Source: CAD feature listing. Evaluate the final solid. Frame: model axes, mm. A direction names the side the tool comes from. Coordinates: 2 decimals unless noted, no trailing zeros. Write each loop counter-clockwise with the first axis right and the second up, starting at its lowest first coordinate (ties: lowest second). Pieces come first, ordered by that corner, then holes. Notation, with made-up numbers: M -31.75,27.25 L 9.25,27.25 A17 cw 9.25,52.25 Z; hole C 66.25,-40 d6. An arc over 180 degrees is marked long. Write item = value, one per line. Start each with the question number.
1. Pull-direction query (X, two-part tool) for faces 4 (the face through (-110, 4, 2)), 5 (the face through (102, 16, 2)), 6 (the face through (77.5, 72, 2)), 7 (the face through (87.5, 72, 2)); classes: pulls with the +X half, pulls with the -X half, needs draft (parallel to the pull), parting line crosses it, or undercut.
2. Access query for faces 1 (the face through (-110, 71, 2)), 2 (the face through (17.5, -2, 2)), 3 (the face through (-35, 70, 2)). Directions: +Z, -Z, +X, -X, +Y, -Y. A direction counts if a zero-diameter tool reaches every point of the face in a straight line with its end or side. Return the directions, or none.
3. Pin query (flat end, axial travel): pin 1 Ø2.5 at (y, z) = (-3.5, 1.5) entering from -X; pin 2 Ø1.5 at (y, z) = (30.5, 2) entering from -X; pin 3 Ø1.5 at (x, z) = (-83, 0.5) entering from -Y; pin 4 Ø12 at (x, y) = (-53, 52.5) entering from -Z. Return the tip coordinate at first contact, or that it passes through.
4. Line query: line 1 along X through (y, z) = (4, 4.45); line 2 along X through (y, z) = (55, 3); line 3 along Y through (x, z) = (82.5, 2.05). Output: solid intervals per line, ascending.
5. Section query A-A (x = 4). Output: boundary loops of the cut face in (y, z).
6. Section query B-B (z = 1.75). Give the number of separate pieces and of enclosed holes in the cut face, then the cut area to 3 significant figures.
```python
from build123d import *

# Parameters (mm, degrees)
SKETCH1_W           = 5
SKETCH1_H           = 5
SKETCH1_R           = 1.5
BOSS_EXTRUDE2_DEPTH = 5


with BuildPart() as part:
    # Sketch1 → Boss-Extrude2 (new body)
    with BuildSketch(Plane.XY):
        Polygon((-110, 80), (-110, 62.5), (-115, 62.5), (-115, 57.5), (-110, 57.5), (-110, 54), (-107, 54), (-107, 55.1), (-104.7, 55.1), (-104.7, 54), (-100, 54), (-100, 51), (-104.7, 51), (-104.7, 49.9), (-107, 49.9), (-107, 51), (-110, 51), (-110, 47.5), (-115, 47.5), (-115, 42.5), (-110, 42.5), (-110, 27.5), (-115, 27.5), (-115, 22.5), (-110, 22.5), (-110, 19), (-107, 19), (-107, 20.1), (-104.7, 20.1), (-104.7, 19), (-100, 19), (-100, 16), (-104.7, 16), (-104.7, 14.9), (-107, 14.9), (-107, 16), (-110, 16), (-110, 12.5), (-115, 12.5), (-115, 7.5), (-110, 7.5), (-110, 0), (-92.5, 0), (-92.5, -5), (-87.5, -5), (-87.5, 0), (-84, 0), (-84, 3), (-85.1, 3), (-85.1, 5.3), (-84, 5.3), (-84, 10), (-81, 10), (-81, 5.3), (-79.9, 5.3), (-79.9, 3), (-81, 3), (-81, 0), (-77.5, 0), (-77.5, -5), (-72.5, -5), (-72.5, 0), (-37.5, 0), (-37.5, -5), (-32.5, -5), (-32.5, 0), (-29, 0), (-29, 3), (-30.1, 3), (-30.1, 5.3), (-29, 5.3), (-29, 10), (-26, 10), (-26, 5.3), (-24.9, 5.3), (-24.9, 3), (-26, 3), (-26, 0), (-22.5, 0), (-22.5, -5), (-17.5, -5), (-17.5, 0), (17.5, 0), (17.5, -5), (22.5, -5), (22.5, 0), (26, 0), (26, 3), (24.9, 3), (24.9, 5.3), (26, 5.3), (26, 10), (29, 10), (29, 5.3), (30.1, 5.3), (30.1, 3), (29, 3), (29, 0), (32.5, 0), (32.5, -5), (37.5, -5), (37.5, 0), (72.5, 0), (72.5, -5), (77.5, -5), (77.5, 0), (81, 0), (81, 3), (79.9, 3), (79.9, 5.3), (81, 5.3), (81, 10), (84, 10), (84, 5.3), (85.1, 5.3), (85.1, 3), (84, 3), (84, 0), (87.5, 0), (87.5, -5), (92.5, -5), (92.5, 0), (110, 0), (110, 7.5), (115, 7.5), (115, 12.5), (110, 12.5), (110, 16), (107, 16), (107, 14.9), (104.7, 14.9), (104.7, 16), (100, 16), (100, 19), (104.7, 19), (104.7, 20.1), (107, 20.1), (107, 19), (110, 19), (110, 22.5), (115, 22.5), (115, 27.5), (110, 27.5), (110, 42.5), (115, 42.5), (115, 47.5), (110, 47.5), (110, 51), (107, 51), (107, 49.9), (104.7, 49.9), (104.7, 51), (100, 51), (100, 54), (104.7, 54), (104.7, 55.1), (107, 55.1), (107, 54), (110, 54), (110, 57.5), (115, 57.5), (115, 62.5), (110, 62.5), (110, 80), align=None)
        with Locations((-90, 72.5)):
            Rectangle(SKETCH1_W, SKETCH1_H, mode=Mode.SUBTRACT)
        with Locations((-82.5, 72.5)):
            Circle(SKETCH1_R, mode=Mode.SUBTRACT)
        with Locations((-75, 72.5)):
            Rectangle(SKETCH1_W, SKETCH1_H, mode=Mode.SUBTRACT)
        with Locations((-35, 72.5)):
            Rectangle(SKETCH1_W, SKETCH1_H, mode=Mode.SUBTRACT)
        with Locations((-27.5, 72.5)):
            Circle(SKETCH1_R, mode=Mode.SUBTRACT)
        with Locations((-20, 72.5)):
            Rectangle(SKETCH1_W, SKETCH1_H, mode=Mode.SUBTRACT)
        with Locations((20, 72.5)):
            Rectangle(SKETCH1_W, SKETCH1_H, mode=Mode.SUBTRACT)
        with Locations((27.5, 72.5)):
            Circle(SKETCH1_R, mode=Mode.SUBTRACT)
        with Locations((35, 72.5)):
            Rectangle(SKETCH1_W, SKETCH1_H, mode=Mode.SUBTRACT)
        with Locations((75, 72.5)):
            Rectangle(SKETCH1_W, SKETCH1_H, mode=Mode.SUBTRACT)
        with Locations((82.5, 72.5)):
            Circle(SKETCH1_R, mode=Mode.SUBTRACT)
        with Locations((90, 72.5)):
            Rectangle(SKETCH1_W, SKETCH1_H, mode=Mode.SUBTRACT)
    extrude(amount=BOSS_EXTRUDE2_DEPTH)


solid = part.part
```
Results are:
q1.face_4 = pulls with the -X half
q1.face_5 = needs draft
q1.face_6 = undercut
q1.face_7 = undercut
q2.face_1 = +Z, -Z, -X, +Y
q2.face_2 = +Z, -Z, -Y
q2.face_3 = +Z, -Z
q3.pin_1 = -92.5
q3.pin_2 = -110
q3.pin_3 = 10
q3.pin_4 = 0
q4.line_1 = -110 to -85.1, -79.9 to -30.1, -24.9 to 24.9, 30.1 to 79.9, 85.1 to 110
q4.line_2 = -110 to -107, -104.7 to 104.7, 107 to 110
q4.line_3 = 10 to 71, 74 to 80
q5.outline = M 0,0 L 80,0 L 80,5 L 0,5 Z
q6.separate_pieces = 1
q6.enclosed_holes = 12
q6.area = 17,500 mm^2
